from build123d import *

# Parameters (mm, degrees)
SKETCH4_W           = 65
SKETCH4_H           = 65
BOSS_EXTRUDE2_DEPTH = 45
SKETCH6_W           = 65
SKETCH6_H           = 65
CUT_EXTRUDE2_DEPTH  = 15
SKETCH7_W           = 10
SKETCH7_H           = 20
CUT_EXTRUDE3_DEPTH  = 92.416994223
SKETCH8_W           = 10
SKETCH8_H           = 20
CUT_EXTRUDE4_DEPTH  = 111.666551289
FILLET1_R           = 15


with BuildPart() as part:
    # Sketch4 → Boss-Extrude2 (new body)
    with BuildSketch(Plane(origin=(0, 0, 0), x_dir=(1, 0, 0), z_dir=(0, 1, 0))):
        with Locations((44.940852102, -13.402797658)):
            Rectangle(SKETCH4_W, SKETCH4_H)
    extrude(amount=-BOSS_EXTRUDE2_DEPTH)

    # Sketch5 → Cut-Revolve2 (revolve, cut)
    with BuildSketch(Plane(origin=(0, 0, 0), x_dir=(1, 0, 0), z_dir=(0, 1, 0))):
        with BuildLine():
            Line((24.940852102, -13.402797658), (64.940852102, -13.402797658))
            ThreePointArc((64.940852102, -13.402797658), (44.940852102, 6.597202342), (24.940852102, -13.402797658))
        make_face()
    revolve(axis=Axis((24.940852102, 0, 13.402797658), (1, 0, 0)), mode=Mode.SUBTRACT)

    # Sketch6 → Cut-Extrude2 (cut)
    with BuildSketch(Plane(origin=(0, 0, 0), x_dir=(1, 0, 0), z_dir=(0, 1, 0))):
        with Locations((44.940852102, -13.402797658)):
            Rectangle(SKETCH6_W, SKETCH6_H)
    extrude(amount=-CUT_EXTRUDE2_DEPTH, mode=Mode.SUBTRACT)

    # Sketch7 → Cut-Extrude3 (cut, through all)
    with BuildSketch(Plane.ZY.offset(-12.440852102)):
        with Locations((-9.097202342, -30)):
            Rectangle(SKETCH7_W, SKETCH7_H)
        with Locations((35.902797658, -30)):
            Rectangle(SKETCH7_W, SKETCH7_H)
    extrude(amount=-CUT_EXTRUDE3_DEPTH, mode=Mode.SUBTRACT)

    # Sketch8 → Cut-Extrude4 (cut, through all)
    with BuildSketch(Plane(origin=(0, 0, -19.097202342), x_dir=(-1, 0, 0), z_dir=(0, 0, -1))):
        with Locations((-67.440852102, -30)):
            Rectangle(SKETCH8_W, SKETCH8_H)
        with Locations((-22.440852102, -30)):
            Rectangle(SKETCH8_W, SKETCH8_H)
    extrude(amount=-CUT_EXTRUDE4_DEPTH, mode=Mode.SUBTRACT)

    # Fillet1
    fillet1_edges = [part.edges().sort_by_distance(p)[0] for p in [
        (27.440852102, -30, 30.902797658),
        (27.440852102, -30, -4.097202342),
        (62.440852102, -30, 30.902797658),
        (62.440852102, -30, -4.097202342),
    ]]
    fillet(fillet1_edges, radius=FILLET1_R)


solid = part.part
Geometry: final body of the model. Coordinates: model frame, mm. A direction names the side the tool comes from. Give positions to 0.01 mm unless a question says otherwise; leave off trailing zeros. Loops run counter-clockwise (first coordinate to the right, second up) from the corner with the lowest first, then second, coordinate; pieces in that order, holes last. Notation, with made-up numbers: M 19,64 L 64,64 A14 ccw 64,77 Z; hole C -24.75,-4.5 d2. An arc over 180 degrees is marked long. Put each result on its own line as item: value.
1) Cut plane A-A, the plane z = -7.5. Return the cut outline in (x, y).
Computed values:
outline: M 12.44,-45 L 77.44,-45 L 77.44,-40 L 12.44,-40 Z; M 12.44,-20 L 77.44,-20 L 77.44,-15 L 12.44,-15 Z
2) Cut plane C-C, the plane x = 16.5. Return the cut outline in (y, z).
Computed values:
outline: M -45,-19.1 L -15,-19.1 L -15,45.9 L -45,45.9 Z; hole M -40,-14.1 L -20,-14.1 L -20,-4.1 L -40,-4.1 Z; hole M -40,30.9 L -20,30.9 L -20,40.9 L -40,40.9 Z
3) Mould query, pull axis X, two halves, no side actions, for faces 1 (the flat face through (17.441, -30, 43)), 2 (the flat face through (75, -30, 30.903)), 3 (the flat face through (12.441, -30, 14)). Classes: released by +X, released by -X, zero draft, split by the parting line, or undercut.
Computed values:
face 1: undercut
face 2: zero draft
face 3: released by -X
4) Cut plane B-B, the plane x = 26.5. Return the cut outline in (y, z), plus the area to 3 significant figures.
Computed values:
outline: M -45,-19.1 L -40,-19.1 L -40,45.9 L -45,45.9 Z; M -20,-19.1 L -15,-19.1 L -15,45.9 L -20,45.9 Z
area: 650 mm^2
5) Material intervals for L1, parallel to Z at x = 43, y = -33.25; L2, parallel to X at y = -33.75, z = -14.5; L3, parallel to Y at x = 23, z = -6, sorted ascending. Write a range as from..to.
Computed values:
L1: z = -19.1..-14.1, -4.1..30.9, 40.9..45.9
L2: x = 12.44..17.44, 27.44..62.44, 72.44..77.44
L3: y = -45..-40, -20..-15
6) Cut plane D-D, the plane z = 19. Return the cut outline in (x, y).
Computed values:
outline: M 12.44,-45 L 77.44,-45 L 77.44,-15 L 56.93,-15 A19.2 cw 32.95,-15 L 12.44,-15 Z; hole M 17.44,-40 L 27.76,-40 L 27.76,-20 L 17.44,-20 Z; hole M 62.12,-40 L 72.44,-40 L 72.44,-20 L 62.12,-20 Z
7) Reachability of faces 4 (the flat face through (44, -45, 13)), 5 (the flat face through (75, -30, -14.097)), 6 (the cylindrical face through (57.93, -30.14, 26.625)), 7 (the flat face through (44, -30, -19.097)), 8 (the flat face through (72.441, -30, 13)) from +Z, -Z, +X, -X, +Y, -Y: full face, straight path, thin tool, end or side. Return the list, or none.
Computed values:
face 4: +Z, -Z, +X, -X, -Y
face 5: +X, -X
face 6: none
face 7: -Z, +X, -X, +Y, -Y
face 8: +Z, -Z
